Check sheet for the drawn part. Datum: minimum x, y, z corner. Units: mm. A direction names the side the tool comes from. Give positions to 0.01 mm unless a question says otherwise; leave off trailing zeros. Write each loop counter-clockwise with the first axis right and the second up, starting at its lowest first coordinate (ties: lowest second). Pieces come first, ordered by that corner, then holes. Notation, with made-up numbers: M 42.5,46.25 L 76.5,46.25 A25 ccw 76.5,68.25 Z; hole C 2,47 d3. An arc over 180 degrees is marked long. Use CSV: the item, a comma, the result in double quotes. Start each with the question number.
1. Cross-section at D-D, the plane x = 6. Enter the section's corners in (y, z), and give its area (3 significant figures).
2. Cross-section at A-A, the plane z = 5. Enter the section's corners in (x, y), and give its area (3 significant figures).
3. Depth check by flat-ended pin: P1, Ø2, axis at x = 7.5, y = 32, coming from the +Z side; P2, Ø6, axis at x = 3.5, y = 7.5, coming from the -Z side; P3, Ø2, axis at x = 8.5, y = 10, coming from the +Z side; P4, Ø3.5, axis at x = 6.5, z = 12, coming from the +Y side. Enter the tip coordinate at first touch or a pass-through.
4. Cross-section at B-B, the plane x = 2. Enter the section's corners in (y, z).
5. Cross-section at C-C, the plane y = 10. Enter the section's corners in (x, z).
6. Access from +Z, -Z, +X, -X, +Y, -Y to the whole of each face (thin tool, end or side, straight path). Record for the marked faces 1, 2 and 3.
7. Scan lines: line 1 (Z direction, x = 8, y = 11.5); line 2 (Y direction, x = 3.5, z = 15.75); line 3 (Y direction, x = 1.5, z = 2.75). Record each from-to range of solid material in increasing order.
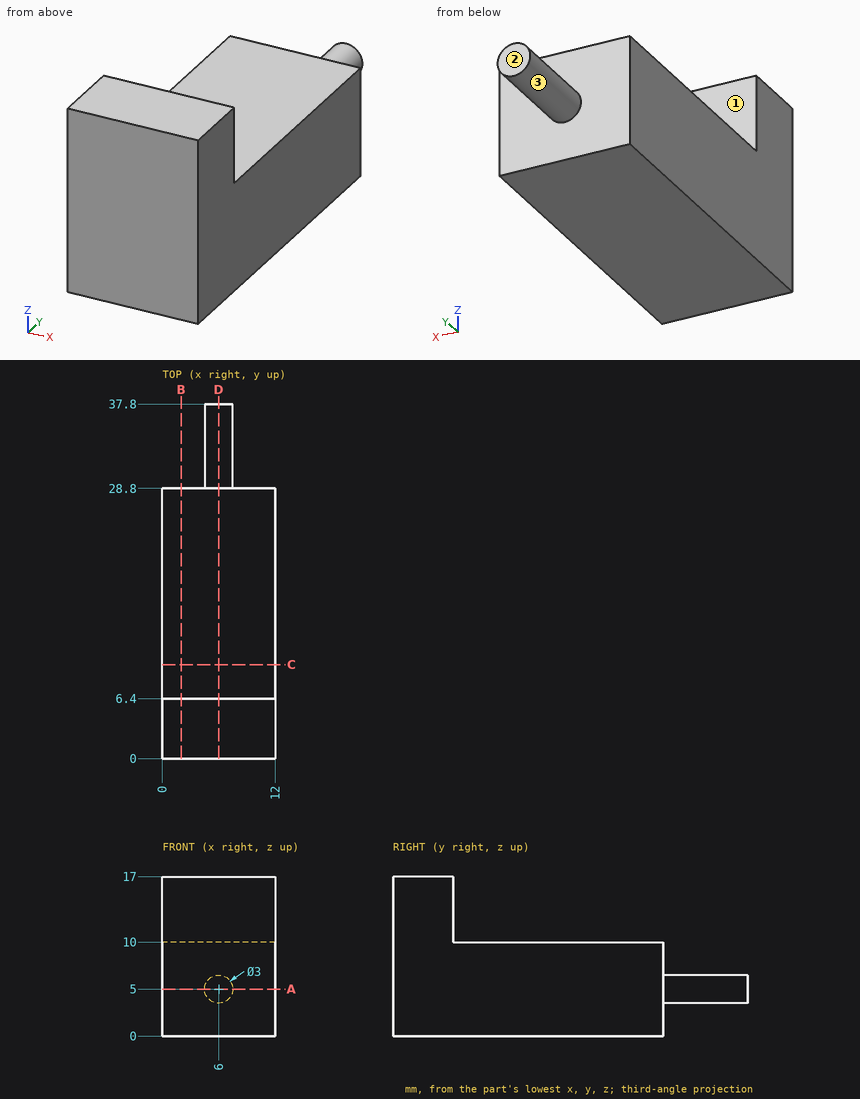
Worked answers:
1,outline,"M 0,0 L 28.8,0 L 28.8,3.5 L 37.8,3.5 L 37.8,6.5 L 28.8,6.5 L 28.8,10 L 6.4,10 L 6.4,17 L 0,17 Z"
1,area,"360 mm^2"
2,outline,"M 0,0 L 12,0 L 12,28.8 L 7.5,28.8 L 7.5,37.8 L 4.5,37.8 L 4.5,28.8 L 0,28.8 Z"
2,area,"373 mm^2"
3,P1,"stops at z = 6.41"
3,P2,"stops at z = 0"
3,P3,"stops at z = 10"
3,P4,"stops at y = 6.4"
4,outline,"M 0,0 L 28.8,0 L 28.8,10 L 6.4,10 L 6.4,17 L 0,17 Z"
5,outline,"M 0,0 L 12,0 L 12,10 L 0,10 Z"
6,face 1,"+Z, +X, -X, +Y"
6,face 2,"+Z, -Z, +X, -X, +Y"
6,face 3,"+Y"
7,line 1,"z = 0 to 10"
7,line 2,"y = 0 to 6.4"
7,line 3,"y = 0 to 28.8"
